Check sheet for the modelled part. Datum: model origin and axes. Units: mm. Face numbers are marked on the shaded views. A direction names the side the tool comes from. Coordinates: 2 decimals unless noted, no trailing zeros. Loops run counter-clockwise (first coordinate to the right, second up) from the corner with the lowest first, then second, coordinate; pieces in that order, holes last. Notation, with made-up numbers: M 85,50 L 98,50 A21 cw 98,55 Z; hole C 28.25,-33.5 d9. An arc over 180 degrees is marked long. Return JSON: item names as keys, results as strings.
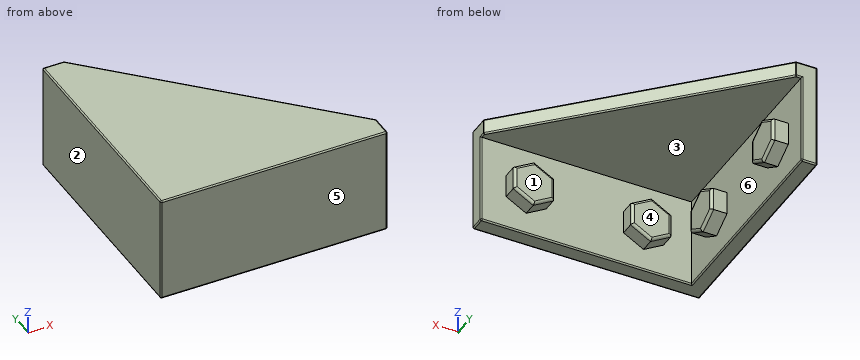
from build123d import *

# Parameters (mm, degrees)
F1_DEPTH = 6
F3_DEPTH = 34
F4_R     = 0.5
F7_DEPTH = 6
F8_R     = 1


# Not quite as in the source:
# - a pattern or mirror of a feature is missing from the dataset's text; its kind, count and spacing are read off the source's solid


with BuildPart() as f1:
    # F0 (on Top) → F1 (new body)
    with BuildSketch(Plane.XY):
        Polygon((0, 85), (0, 0), (85, 0), (85, 8), (8, 85), align=None)
    extrude(amount=F1_DEPTH)

    # F2 (on Top) → F3 (join)
    with BuildSketch(Plane.XY):
        Polygon((0, 85), (0, 0), (85, 0), (85, 6), (6, 6), (6, 85), align=None)
    extrude(amount=-F3_DEPTH)

    # F4
    f4_edges = [f1.edges().sort_by_distance(p)[0] for p in [
        (0, 42.5, -34),
        (42.5, 0, -34),
        (85, 3, -34),
        (45.5, 6, -34),
        (6, 45.5, -34),
        (3, 85, -34),
        (0, 85, -14),
        (0, 42.5, 6),
        (0, 0, -14),
        (8, 85, 3),
        (4, 85, 6),
        (6, 85, -17),
        (7, 85, 0),
        (85, 8, 3),
        (46.5, 46.5, 0),
        (46.5, 46.5, 6),
        (42.5, 0, 6),
        (85, 4, 6),
        (85, 0, -14),
        (85, 7, 0),
        (85, 6, -17),
    ]]
    fillet(f4_edges, radius=F4_R)

    # F6 (on face) → F7 (join)
    with BuildSketch(Plane(origin=(0, 6, 0), x_dir=(-1, 0, 0), z_dir=(0, 1, 0))):
        Polygon((-68, -25.6602540378), (-60.5, -21.3301270189), (-60.5, -12.6698729811), (-68, -8.3397459622), (-75.5, -12.6698729811), (-75.5, -21.3301270189), align=None)
        Polygon((-24, -25.6602540378), (-16.5, -21.3301270189), (-16.5, -12.6698729811), (-24, -8.3397459622), (-31.5, -12.6698729811), (-31.5, -21.3301270189), align=None)
    f7 = extrude(amount=F7_DEPTH)

    # F7_copies: F7 across plane
    add(f7.mirror(Plane(origin=(0, 0, 0), x_dir=(0.7071067812, 0.7071067812, 0), z_dir=(-0.7071067812, 0.7071067812, 0))))

    # F8
    f8_edges = [f1.edges().sort_by_distance(p)[0] for p in [
        (71.75, 12, -23.495191),
        (64.25, 12, -23.495191),
        (60.5, 12, -17),
        (64.25, 12, -10.504809),
        (71.75, 12, -10.504809),
        (75.5, 12, -17),
        (27.75, 12, -23.495191),
        (20.25, 12, -23.495191),
        (16.5, 12, -17),
        (20.25, 12, -10.504809),
        (27.75, 12, -10.504809),
        (31.5, 12, -17),
        (12, 31.5, -17),
        (12, 27.75, -10.504809),
        (12, 20.25, -10.504809),
        (12, 16.5, -17),
        (12, 20.25, -23.495191),
        (12, 27.75, -23.495191),
        (12, 75.5, -17),
        (12, 71.75, -10.504809),
        (12, 64.25, -10.504809),
        (12, 60.5, -17),
        (12, 64.25, -23.495191),
        (12, 71.75, -23.495191),
    ]]
    fillet(f8_edges, radius=F8_R)


solid = f1.part
1) Section check A-A on z = -3.5. Record the cut outline in (x, y), then the cut area to 3 significant figures.
Answers:
{"outline": "M 0,0.5 A0.5 ccw 0.5,0 L 84.5,0 A0.5 ccw 85,0.5 L 85,5.5 A0.5 ccw 84.5,6 L 6,6 L 6,84.5 A0.5 ccw 5.5,85 L 0.5,85 A0.5 ccw 0,84.5 Z", "area": "984 mm²"}
2) Scan lines: line 1 along Y through (x, z) = (36, -25); line 2 along X through (y, z) = (9, -10). Record each from-to range of solid material in increasing order. Write a range as [from, to].
Answers:
{"line 1": "[0, 6]", "line 2": "[0, 6], [21.12, 26.88], [65.12, 70.88]"}
3) Set-up check for the marked faces 1 and 2: record each of +Z, -Z, +X, -X, +Y, -Y from which the full face is reachable in a straight line by a thin tool's end or side.
Answers:
{"face 1": "-Z, +X, +Y", "face 2": "+Z, -Z, -X, +Y, -Y"}
4) Draft check along Y on the marked faces 3, 4, 5 and 6. Enter one of: +Y half, -Y half, draft (parallel to the pull), parting line (faces both ways), or undercut.
Answers:
{"face 3": "draft", "face 4": "+Y half", "face 5": "-Y half", "face 6": "undercut"}
5) Go/stop test with flat-tipped pins: pin 1 Ø8 at (y, z) = (47.5, -6.5) entering from +X; pin 2 Ø6.5 at (y, z) = (21, -19.5) entering from +X; pin 3 Ø4 at (y, z) = (8.5, -15.5) entering from +X. Record where each tip stops, or that it passes through.
Answers:
{"pin 1": "x = 6", "pin 2": "x = 12", "pin 3": "x = 75.5"}
